from build123d import *

# Parameters (mm, degrees)
BOSS_EXTRUDE1_DEPTH = 16.5
SKETCH5_R           = 1.5
CUT_EXTRUDE1_DEPTH  = 34
SKETCH2_R           = 2.5
BOSS_EXTRUDE2_DEPTH = 24
SKETCH3_R           = 11
BOSS_EXTRUDE3_DEPTH = 2


with BuildPart() as part:
    # Sketch1 → Boss-Extrude1 (new body, symmetric)
    with BuildSketch(Plane.XY):
        with BuildLine():
            Line((-16.15, -21.15), (16.15, -21.15))
            ThreePointArc((16.15, -21.15), (19.685533906, -19.685533906), (21.15, -16.15))
            Line((21.15, -16.15), (21.15, 16.15))
            ThreePointArc((21.15, 16.15), (19.685533906, 19.685533906), (16.15, 21.15))
            Line((16.15, 21.15), (-16.15, 21.15))
            ThreePointArc((-16.15, 21.15), (-19.685533906, 19.685533906), (-21.15, 16.15))
            Line((-21.15, 16.15), (-21.15, -16.15))
            ThreePointArc((-21.15, -16.15), (-19.685533906, -19.685533906), (-16.15, -21.15))
        make_face()
    extrude(amount=BOSS_EXTRUDE1_DEPTH, both=True)

    # Sketch5 → Cut-Extrude1 (cut, through all)
    with BuildSketch(Plane.XY.offset(16.5)):
        with Locations((-15.5, 15.5)):
            Circle(SKETCH5_R)
        with Locations((15.5, 15.5)):
            Circle(SKETCH5_R)
        with Locations((15.5, -15.5)):
            Circle(SKETCH5_R)
        with Locations((-15.5, -15.5)):
            Circle(SKETCH5_R)
    extrude(amount=-CUT_EXTRUDE1_DEPTH, mode=Mode.SUBTRACT)

    # Sketch2 → Boss-Extrude2 (add)
    with BuildSketch(Plane.XY.offset(16.5)):
        Circle(SKETCH2_R)
    extrude(amount=BOSS_EXTRUDE2_DEPTH)

    # Sketch3 → Boss-Extrude3 (add)
    with BuildSketch(Plane.XY.offset(16.5)):
        Circle(SKETCH3_R)
    extrude(amount=BOSS_EXTRUDE3_DEPTH)


solid = part.part
The model under review builds one solid part; all positions refer to its coordinate system, in mm. A direction names the side the tool comes from. Round coordinates to 2 decimals unless told otherwise and drop trailing zeros. Order: outer loops, then holes, each group sorted by start corner. A loop starts at its lowest first (then second) coordinate and runs counter-clockwise, first axis right, second up. Notation, with made-up numbers: (60.5, 5) -> (93.5, 5) arc R12 ccw to (93.5, 21) -> close; hole circle Ø7 at (48.25, 2). An arc over 180 degrees is marked (long way). Return JSON: item names as keys, results as strings.
1. For faces 4 (the face through (-10, -9, 16.5)), 5 (the face through (-21.15, 0, 0)), list the 3-axis set-ups (+Z, -Z, +X, -X, +Y, -Y) from which the entire face can be reached by the end or side of a thin tool; tool diameter is ignored.
Answer block:
{"face 4": "+Z", "face 5": "+Z, -Z, -X, +Y, -Y"}
2. Take a section at A-A (z = 10.5). Write out the cut boundary in (x, y).
Answer block:
{"outline": "(-21.15, -16.15) arc R5 ccw to (-16.15, -21.15) -> (16.15, -21.15) arc R5 ccw to (21.15, -16.15) -> (21.15, 16.15) arc R5 ccw to (16.15, 21.15) -> (-16.15, 21.15) arc R5 ccw to (-21.15, 16.15) -> close; hole circle Ø3 at (-15.5, -15.5); hole circle Ø3 at (-15.5, 15.5); hole circle Ø3 at (15.5, -15.5); hole circle Ø3 at (15.5, 15.5)"}
3. For L1, parallel to Y at x = 15.5, z = -6.5; L2, parallel to X at y = 15, z = -9; L3, parallel to Z at x = -5, y = -11.5, list the stretches that pass through material, from the lowest coordinate up. Write a range as [from, to].
Answer block:
{"L1": "y = [-21.15, -17], [-14, 14], [17, 21.15]", "L2": "x = [-21.15, -16.91], [-14.09, 14.09], [16.91, 21.15]", "L3": "z = [-16.5, 16.5]"}
4. Insertion check: P1, Ø2.5, axis at x = -15.5, y = 15.5, coming from the -Z side; P2, Ø2, axis at x = 0, z = 27.5, coming from the +Y side; P3, Ø21, axis at x = 2.5, y = 7, coming from the +Z side; P4, Ø2, axis at x = -13, y = 4.5, coming from the +Z side. Each pin has a flat end and moves straight along its axis. Give the tip position at first contact, or say it passes through.
Answer block:
{"P1": "passes through", "P2": "stops at y = 2.5", "P3": "stops at z = 40.5", "P4": "stops at z = 16.5"}
5. Take a section at D-D (x = -1). Write out the cut boundary in (y, z), then the cut area to 3 significant figures.
Answer block:
{"outline": "(-21.15, -16.5) -> (21.15, -16.5) -> (21.15, 16.5) -> (10.95, 16.5) -> (10.95, 18.5) -> (2.29, 18.5) -> (2.29, 40.5) -> (-2.29, 40.5) -> (-2.29, 18.5) -> (-10.95, 18.5) -> (-10.95, 16.5) -> (-21.15, 16.5) -> close", "area": "1,540 mm²"}
6. Take a section at B-B (x = -15). Write out the cut boundary in (y, z).
Answer block:
{"outline": "(-21.15, -16.5) -> (-16.91, -16.5) -> (-16.91, 16.5) -> (-21.15, 16.5) -> close; (-14.09, -16.5) -> (14.09, -16.5) -> (14.09, 16.5) -> (-14.09, 16.5) -> close; (16.91, -16.5) -> (21.15, -16.5) -> (21.15, 16.5) -> (16.91, 16.5) -> close"}
7. Take a section at C-C (y = 0). Write out the cut boundary in (x, z), then the cut area to 3 significant figures.
Answer block:
{"outline": "(-21.15, -16.5) -> (21.15, -16.5) -> (21.15, 16.5) -> (11, 16.5) -> (11, 18.5) -> (2.5, 18.5) -> (2.5, 40.5) -> (-2.5, 40.5) -> (-2.5, 18.5) -> (-11, 18.5) -> (-11, 16.5) -> (-21.15, 16.5) -> close", "area": "1,550 mm²"}
8. The part is to be moulded in two halves that separate along X. For faces 1 (the face through (-17, -15.43, 0.23)), 2 (the face through (0, 0, -16.5)), 3 (the face through (-0.54, -2.44, 29.35)), say which applies: +X half, -X half, draft (parallel to the pull), parting line (faces both ways), or undercut.
Answer block:
{"face 1": "undercut", "face 2": "draft", "face 3": "parting line"}
